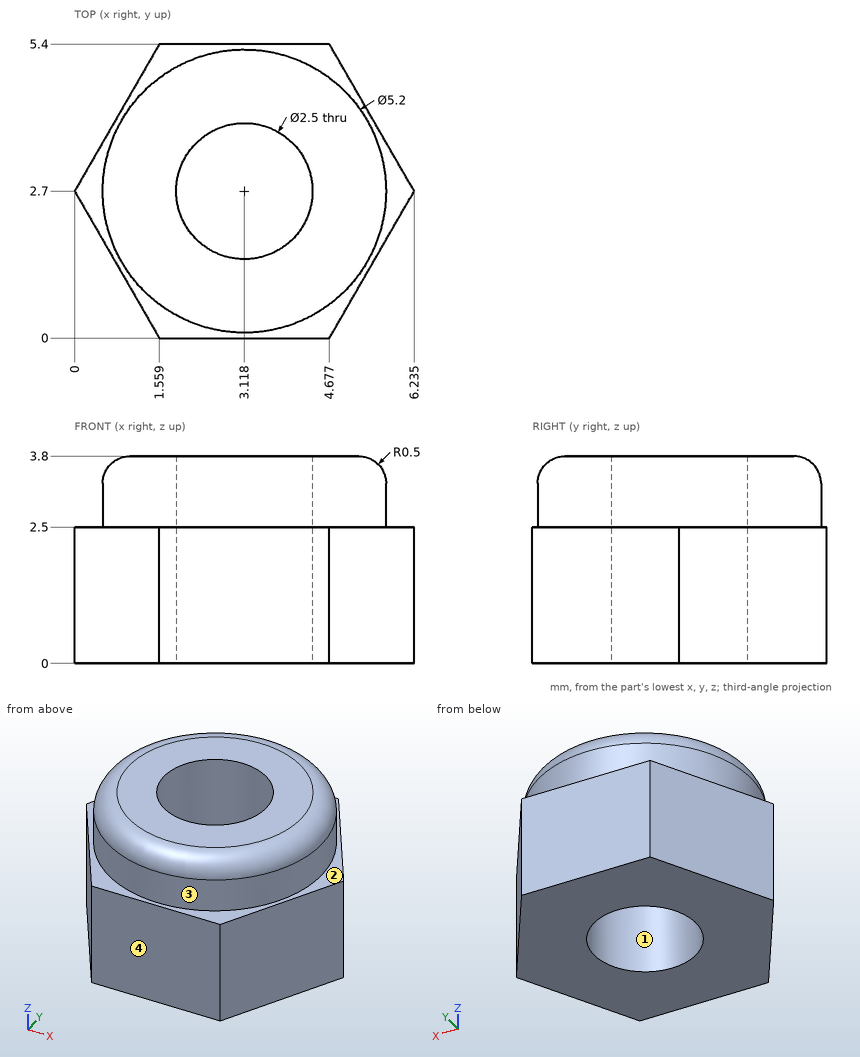
Geometry: see drawing. Coordinates: mm, zero at the bounding-box minimum. Coordinates: 2 decimals unless noted, no trailing zeros. Answer in a Markdown table with one row per item. Add a question column.
Q1. Contact query for a flat-ended pin moving along its axis: P1, Ø3, axis at x = 3.12, y = 2.7, coming from the +Z side. Output: stop coordinate, or through.
Q2. Line query: L1, parallel to X at y = 2.7, z = 3.05; L2, parallel to Z at x = 1.5, y = 0.45; L3, parallel to Z at x = 1.5, y = 4.1. Output: solid intervals per line, ascending.
Q3. Mould query, pull axis Y, two halves, no side actions, for the marked faces 1, 2, 3 and 4. Classes: released by +Y, released by -Y, zero draft, split by the parting line, or undercut.
Completed:
| question | item | result |
|---|---|---|
| 1 | P1 | stops at z = 3.8 |
| 2 | L1 | x = 0.52 to 1.87, 4.37 to 5.72 |
| 2 | L2 | z = 0 to 2.5 |
| 2 | L3 | z = 0 to 3.8 |
| 3 | face 1 | undercut |
| 3 | face 2 | zero draft |
| 3 | face 3 | split by the parting line |
| 3 | face 4 | released by -Y |
